Check sheet for the modelled part. Datum: model origin and axes. Units: mm. Round coordinates to 2 decimals unless told otherwise and drop trailing zeros. Order: outer loops, then holes, each group sorted by start corner. A loop starts at its lowest first (then second) coordinate and runs counter-clockwise, first axis right, second up.
(1) Sectioned sample at D-D, the plane z = -51. Enter the section's corners in (x, y), and give its area (3 significant figures).
(2) Sectioned sample at C-C, the plane y = 6. Enter the section's corners in (x, z).
(3) Sectioned sample at A-A, the plane z = -10. Enter the section's corners in (x, y) (3 decimals).
(4) Sectioned sample at B-B, the plane x = 0. Count the separate pieces of the cut face and the enclosed holes in it, and give its area (3 significant figures).
(5) Thickness scan on probe 1 along Y at (x, z) = (5.75, -62); probe 2 along X at (y, z) = (-9.1, -10) (3 decimals). Record the ranges inside material, lowest first.
(6) Depth check by flat-ended pin: pin 1 (5.5 mm diameter, centred on x = 0, z = -80, fed in from -Y); pin 2 (2.5 mm diameter, centred on x = 0, z = -150, fed in from -Y). Enter the tip coordinate at first touch or a pass-through.
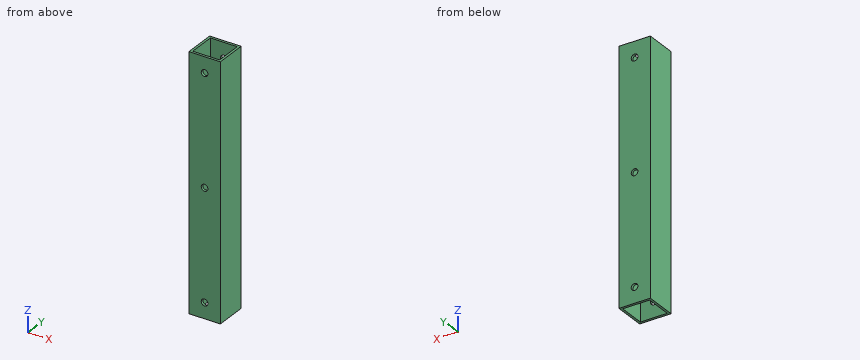
```python
from build123d import *

# Parameters (mm, degrees)
SKETCH1_W           = 20
SKETCH1_H           = 20
SKETCH1_W_2         = 17
SKETCH1_H_2         = 17
BOSS_EXTRUDE1_DEPTH = 160
SKETCH2_R           = 2.125
CUT_EXTRUDE1_DEPTH  = 162.554944214


with BuildPart() as part:
    # Sketch1 → Boss-Extrude1 (new body)
    with BuildSketch(Plane.XY):
        Rectangle(SKETCH1_W, SKETCH1_H)
        Rectangle(SKETCH1_W_2, SKETCH1_H_2, mode=Mode.SUBTRACT)
    extrude(amount=-BOSS_EXTRUDE1_DEPTH)

    # Sketch2 → Cut-Extrude1 (cut, through all)
    with BuildSketch(Plane(origin=(0, 10, 0), x_dir=(1, 0, 0), z_dir=(0, 1, 0))):
        with Locations(Location((0, 10, 0), (0, 0, 270))):
            Circle(SKETCH2_R)
        with Locations(Location((0, 80, 0), (0, 0, 270))):
            Circle(SKETCH2_R)
        with Locations(Location((0, 150, 0), (0, 0, 270))):
            Circle(SKETCH2_R)
    extrude(amount=-CUT_EXTRUDE1_DEPTH, mode=Mode.SUBTRACT)


solid = part.part
```
Derived:
1. outline: (-10, -10) - (10, -10) - (10, 10) - (-10, 10) - close; hole (-8.5, -8.5) - (8.5, -8.5) - (8.5, 8.5) - (-8.5, 8.5) - close
1. area: 111 mm2
2. outline: (-10, -160) - (-8.5, -160) - (-8.5, 0) - (-10, 0) - close; (8.5, -160) - (10, -160) - (10, 0) - (8.5, 0) - close
3. outline: (-10, -10) - (-2.125, -10) - (-2.125, -8.5) - (-8.5, -8.5) - (-8.5, 8.5) - (-2.125, 8.5) - (-2.125, 10) - (-10, 10) - close; (2.125, -10) - (10, -10) - (10, 10) - (2.125, 10) - (2.125, 8.5) - (8.5, 8.5) - (8.5, -8.5) - (2.125, -8.5) - close
4. separate pieces: 8
4. enclosed holes: 0
4. area: 442 mm2
5. probe 1: y = -10 to -8.5, 8.5 to 10
5. probe 2: x = -10 to -2.125, 2.125 to 10
6. pin 1: stops at y = -10
6. pin 2: passes through
